Read the model definition and answer for the solid it produces. Units are mm, in the model's axes. Coordinates: 2 decimals unless noted, no trailing zeros. Loops run counter-clockwise (first coordinate to the right, second up) from the corner with the lowest first, then second, coordinate; pieces in that order, holes last.
Q1. Flat-ended cylindrical pins translate along their axes: P1, Ø1, axis at x = 62, z = 2, coming from the +Y side; P2, Ø1.9, axis at y = 21, z = 2.5, coming from the +X side; P3, Ø3, axis at y = 44, z = 5.5, coming from the +X side. Find the tip coordinate at first contact, or state that the pin passes through.
Q2. The mould has two halves that part along Z. Classify faces 1 (the face through (283, 26, 0)), 2 (the face through (283, 26, 6.35)): pulls with the +Z half, pulls with the -Z half, needs draft (parallel to the pull), parting line crosses it, or undercut.
Q3. Section C-C (x = 467) is taken. Give the vertices of the cut face in (y, z).
Q4. Straight lines are drawn through the part: line 1 (Y direction, x = 101.6, z = 3.5); line 2 (X direction, y = -18.5, z = 4.25); line 3 (Y direction, x = 202, z = 4). For each, find the intervals that lie inside material, in ascending order.
Q5. Section B-B (x = 167) is taken. Give the vertices of the cut face in (y, z), then the cut area to 3 significant figures.
Q6. Section A-A (z = 4) is taken. Count the separate pieces of the cut face and the enclosed holes in it, then the cut area to 3 significant figures.
from build123d import *

# Parameters (mm, degrees)
SKETCH1_R           = 4.127
SKETCH1_R_2         = 4
SKETCH1_R_3         = 2.4892
BOSS_EXTRUDE1_DEPTH = 6.35


with BuildPart() as part:
    # Sketch1 → Boss-Extrude1 (new body)
    with BuildSketch(Plane.XY):
        with BuildLine():
            Line((0, 50.8), (69.782797106, 50.8))
            ThreePointArc((69.782797106, 50.8), (79.63302553, 54.01434095), (85.691398553, 62.42))
            ThreePointArc((85.691398553, 62.42), (101.6, 74.04), (117.508601447, 62.42))
            ThreePointArc((117.508601447, 62.42), (123.56697447, 54.01434095), (133.417202894, 50.8))
            Line((133.417202894, 50.8), (459.482797106, 50.8))
            ThreePointArc((459.482797106, 50.8), (469.33302553, 54.01434095), (475.391398553, 62.42))
            ThreePointArc((475.391398553, 62.42), (488.001405867, 73.710988875), (504, 68.184353369))
            ThreePointArc((504, 68.184353369), (516.7, 62.328706739), (529.4, 68.184353369))
            ThreePointArc((529.4, 68.184353369), (551.811441752, 70.92594491), (556.471129688, 48.833494754))
            ThreePointArc((556.471129688, 48.833494754), (553.958009173, 42.90331161), (553.1, 36.52))
            Line((553.1, 36.52), (515.860000058, 36.52))
            Line((515.860000058, 36.52), (515.860000058, 14.28))
            Line((515.860000058, 14.28), (553.1, 14.28))
            ThreePointArc((553.1, 14.28), (553.958009173, 7.89668839), (556.471129688, 1.966505246))
            ThreePointArc((556.471129688, 1.966505246), (551.811441752, -20.12594491), (529.4, -17.384353369))
            ThreePointArc((529.4, -17.384353369), (516.7, -11.528706739), (504, -17.384353369))
            ThreePointArc((504, -17.384353369), (488.001405867, -22.910988875), (475.391398553, -11.62))
            ThreePointArc((475.391398553, -11.62), (469.33302553, -3.21434095), (459.482797106, 0))
            Line((459.482797106, 0), (133.417202894, 0))
            ThreePointArc((133.417202894, 0), (123.56697447, -3.21434095), (117.508601447, -11.62))
            ThreePointArc((117.508601447, -11.62), (101.6, -23.24), (85.691398553, -11.62))
            ThreePointArc((85.691398553, -11.62), (79.63302553, -3.21434095), (69.782797106, 0))
            Line((69.782797106, 0), (0, 0))
            Line((0, 0), (0, 50.8))
        make_face()
        with Locations((13.54, 38.94)):
            Circle(SKETCH1_R, mode=Mode.SUBTRACT)
        with Locations(Location((101.6, -6.54, 0), (0, 0, 180))):
            Circle(SKETCH1_R_2, mode=Mode.SUBTRACT)
        with Locations((481.98, 13.3425)):
            Circle(SKETCH1_R_3, mode=Mode.SUBTRACT)
        with Locations((481.98, 37.4575)):
            Circle(SKETCH1_R_3, mode=Mode.SUBTRACT)
        with Locations((276.55, 13.3425)):
            Circle(SKETCH1_R_3, mode=Mode.SUBTRACT)
        with Locations((71.12, 13.3425)):
            Circle(SKETCH1_R_3, mode=Mode.SUBTRACT)
        with Locations((71.12, 37.4575)):
            Circle(SKETCH1_R_3, mode=Mode.SUBTRACT)
        with Locations((101.6, 57.34)):
            Circle(SKETCH1_R_2, mode=Mode.SUBTRACT)
        with Locations((491.3, 57.34)):
            Circle(SKETCH1_R_2, mode=Mode.SUBTRACT)
        with Locations((542.1, 57.34)):
            Circle(SKETCH1_R_2, mode=Mode.SUBTRACT)
        with Locations(Location((542.1, -6.54, 0), (0, 0, 180))):
            Circle(SKETCH1_R_2, mode=Mode.SUBTRACT)
        with Locations(Location((491.3, -6.54, 0), (0, 0, 180))):
            Circle(SKETCH1_R_2, mode=Mode.SUBTRACT)
    extrude(amount=BOSS_EXTRUDE1_DEPTH)


solid = part.part
Numbers:
1. P1: stops at y = 50.8
1. P2: stops at x = 515.86
1. P3: stops at x = 554.83
2. face 1: pulls with the -Z half
2. face 2: pulls with the +Z half
3. outline: (-1.79, 0) - (52.59, 0) - (52.59, 6.35) - (-1.79, 6.35) - close
4. line 1: y = -23.24 to -10.54, -2.54 to 53.34, 61.34 to 74.04
4. line 2: x = 89.94 to 113.26, 479.64 to 502.96, 530.44 to 553.76
4. line 3: y = 0 to 50.8
5. outline: (0, 0) - (50.8, 0) - (50.8, 6.35) - (0, 6.35) - close
5. area: 323 mm2
6. separate pieces: 1
6. enclosed holes: 12
6. area: 31,500 mm2
